from build123d import *

# Parameters (mm, degrees)
F0_W      = 44.5
F0_H      = 110
F0_R      = 2.65
F1_DEPTH  = 4
F2_W      = 44.5
F2_H      = 4
F3_DEPTH  = 20
F4_W      = 4
F4_H      = 68.5
F4_H_2    = 13.5
F5_DEPTH  = 20
F7_DEPTH  = 20
F9_DEPTH  = 15
F11_DEPTH = 44.501
F12_DEPTH = 20.001
F14_DEPTH = 20
F15_W     = 44.5
F15_H     = 9
F16_DEPTH = 1.5
F17_SIZE  = 1.49999
F18_DEPTH = 20.001
F19_SIZE  = 2


# Not quite as in the source:
# - a fillet or chamfer is up to 0.001 mm smaller than in the source, because OpenCascade refuses the exact size


with BuildPart() as f1:
    # F0 (on Top) → F1 (new body)
    with BuildSketch(Plane.XY):
        with Locations((22.25, 55)):
            Rectangle(F0_W, F0_H)
        with BuildLine():
            Line((25.25, 35), (25.25, 10))
            ThreePointArc((25.25, 10), (22.25, 7), (19.25, 10))
            Line((19.25, 10), (19.25, 35))
            ThreePointArc((19.25, 35), (22.25, 38), (25.25, 35))
        make_face(mode=Mode.SUBTRACT)
        with Locations((10, 100)):
            Circle(F0_R, mode=Mode.SUBTRACT)
        with Locations((22.25, 82.5)):
            Circle(F0_R, mode=Mode.SUBTRACT)
        with Locations((34.5, 100)):
            Circle(F0_R, mode=Mode.SUBTRACT)
    extrude(amount=F1_DEPTH)

    # F2 (on face) → F3 (join)
    with BuildSketch(Plane(origin=(0, 0, 0), x_dir=(1, 0, 0), z_dir=(0, 0, -1))):
        with Locations((22.25, -94.5)):
            Rectangle(F2_W, F2_H)
        with Locations((22.25, -70.5)):
            Rectangle(F2_W, F2_H)
    extrude(amount=F3_DEPTH)

    # F4 (on face) → F5 (join)
    with BuildSketch(Plane(origin=(0, 0, 0), x_dir=(1, 0, 0), z_dir=(0, 0, -1))):
        with Locations((2, -34.25)):
            Rectangle(F4_W, F4_H)
        with Locations((42.5, -34.25)):
            Rectangle(F4_W, F4_H)
        Polygon((0, -96.5), (0, -110), (4, -110), (4, -103.4641016151), (4, -96.5358983849), (4, -96.5), align=None)
        Polygon((4, -96.5358983849), (4, -103.4641016151), (10, -106.9282032303), (16, -103.4641016151), (16, -96.5358983849), (15.9378221735, -96.5), (11.9378221735, -96.5), (14, -97.6905989232), (14, -102.3094010768), (10, -104.6188021535), (6, -102.3094010768), (6, -97.6905989232), (8.0621778265, -96.5), (4.0621778265, -96.5), align=None)
        Polygon((11.9378221735, -96.5), (8.0621778265, -96.5), (6, -97.6905989232), (6, -102.3094010768), (10, -104.6188021535), (14, -102.3094010768), (14, -97.6905989232), align=None)
        Polygon((40.5, -110), (44.5, -110), (44.5, -96.5), (40.5, -96.5), (40.5, -96.5358983849), (40.5, -103.4641016151), align=None)
        Polygon((34.5, -106.9282032303), (40.5, -103.4641016151), (40.5, -96.5358983849), (40.4378221735, -96.5), (36.4378221735, -96.5), (38.5, -97.6905989232), (38.5, -102.3094010768), (34.5, -104.6188021535), (30.5, -102.3094010768), (30.5, -97.6905989232), (32.5621778265, -96.5), (28.5621778265, -96.5), (28.5, -96.5358983849), (28.5, -103.4641016151), align=None)
        Polygon((38.5, -97.6905989232), (36.4378221735, -96.5), (32.5621778265, -96.5), (30.5, -97.6905989232), (30.5, -102.3094010768), (34.5, -104.6188021535), (38.5, -102.3094010768), align=None)
        Polygon((32.5621778265, -96.5), (36.4378221735, -96.5), (34.5, -95.3811978465), align=None)
        with Locations((16.25, -34.25)):
            Rectangle(F4_W, F4_H)
        with Locations((28.25, -34.25)):
            Rectangle(F4_W, F4_H)
        with Locations((22.25, -103.25)):
            Rectangle(F4_W, F4_H_2)
    extrude(amount=F5_DEPTH)

    # F6 (on face) → F7 (join)
    with BuildSketch(Plane(origin=(0, 0, 0), x_dir=(1, 0, 0), z_dir=(0, 0, -1))):
        Polygon((40.5, -96.5), (40.4378221735, -96.5), (40.5, -96.5358983849), align=None)
        Polygon((4.0621778265, -96.5), (4, -96.5), (4, -96.5358983849), align=None)
        Polygon((16, -96.5358983849), (16, -103.4641016151), (20.25, -103.4641016151), (20.25, -96.5), (15.9378221735, -96.5), align=None)
        Polygon((28.5621778265, -96.5), (24.25, -96.5), (24.25, -103.4641016151), (28.5, -103.4641016151), (28.5, -96.5358983849), align=None)
    extrude(amount=F7_DEPTH)

    # F8 (on face) → F9 (cut)
    with BuildSketch(Plane(origin=(0, 0, -20), x_dir=(1, 0, 0), z_dir=(0, 0, -1))):
        Polygon((4, -103.4641016151), (10, -106.9282032303), (16, -103.4641016151), (20.25, -103.4641016151), (20.25, -96.5), (4, -96.5), align=None)
        Polygon((24.25, -103.4641016151), (28.5, -103.4641016151), (34.5, -106.9282032303), (40.5, -103.4641016151), (40.5, -96.5), (24.25, -96.5), align=None)
    extrude(amount=-F9_DEPTH, mode=Mode.SUBTRACT)

    # F10 (on face) → F11 (cut, through all)
    with BuildSketch(Plane(origin=(0, 0, 0), x_dir=(0, -1, 0), z_dir=(-1, 0, 0))):
        Polygon((-96.5, -20), (-110, 0), (-110, -20), align=None)
        Polygon((0, -5), (-68.5, -20), (0, -20), align=None)
    extrude(amount=-F11_DEPTH, mode=Mode.SUBTRACT)

    # F12 (cut, through all): faces of the model
    f12_faces = [f1.faces().sort_by_distance(p)[0] for p in [
        (34.5, 100, 0),
        (10, 100, 0),
    ]]
    extrude(f12_faces, amount=-F12_DEPTH, mode=Mode.SUBTRACT)

    # F13 (on face) → F14 (cut, through all)
    with BuildSketch(Plane(origin=(0, 0, -20), x_dir=(1, 0, 0), z_dir=(0, 0, -1))):
        Polygon((14, -102.3094010768), (14, -97.6905989232), (10, -95.3811978465), (6, -97.6905989232), (6, -102.3094010768), (10, -104.6188021535), align=None)
        Polygon((38.5, -102.3094010768), (38.5, -97.6905989232), (34.5, -95.3811978465), (30.5, -97.6905989232), (30.5, -102.3094010768), (34.5, -104.6188021535), align=None)
    extrude(amount=-F14_DEPTH, mode=Mode.SUBTRACT)

    # F15 (on face) → F16 (join)
    with BuildSketch(Plane(origin=(0, 0, 0), x_dir=(1, 0, 0), z_dir=(0, 0, -1))):
        with Locations((22.25, -82.5)):
            Rectangle(F15_W, F15_H)
    extrude(amount=F16_DEPTH)

    # F17 (size 1.5 in the source; OpenCascade refuses exactly that, so slightly less here)
    f17_edges = [f1.edges().sort_by_distance(p)[0] for p in [
        (44.5, 82.5, -1.5),
        (22.25, 78, -1.5),
        (0, 82.5, -1.5),
        (22.25, 87, -1.5),
    ]]
    chamfer(f17_edges, length=F17_SIZE)

    # F18 (cut, through all): a face of the model
    f18_faces = [f1.faces().sort_by_distance(p)[0] for p in [
        (22.25, 82.5, 0),
    ]]
    extrude(f18_faces, amount=-F18_DEPTH, mode=Mode.SUBTRACT)

    # F19
    f19_edges = [f1.edges().sort_by_distance(p)[0] for p in [
        (44.5, 110, 2),
        (0, 110, 2),
        (0, 0, -0.5),
        (44.5, 0, -0.5),
    ]]
    chamfer(f19_edges, length=F19_SIZE)


solid = f1.part
Check sheet for the modelled part. Datum: model origin and axes. Units: mm. A direction names the side the tool comes from. Give positions to 0.01 mm unless a question says otherwise; leave off trailing zeros. Order: outer loops, then holes, each group sorted by start corner. A loop starts at its lowest first (then second) coordinate and runs counter-clockwise, first axis right, second up. Notation, with made-up numbers: M -6.5,-11 L 47.5,-11 A24 ccw 47.5,6 Z; hole C 47.5,-11.75 d5. An arc over 180 degrees is marked long. Answer as CSV lines item,"result". Start each with the question number.
Item 1: Cross-section at B-B on y = 14.5. Enter the section's corners in (x, z), plus the area to 3 significant figures.
Item 2: Cross-section at A-A on x = 22.25. State how many separate pieces and enclosed holes the cut face has, plus the area to 3 significant figures.
Item 3: Gauge pin test, flat ends, axial feed: P1, Ø11, axis at x = 11.5, y = 103.5, coming from the -Z side; P2, Ø1.5, axis at x = 8, y = 63.5, coming from the -Z side; P3, Ø1.3, axis at x = 26.5, z = -2, coming from the +Y side; P4, Ø8, axis at y = 35, z = -17, coming from the +X side. Record the tip position at first contact, or that the pin passes through.
Item 4: Cross-section at D-D on y = 82.5. Enter the section's corners in (x, z).
Item 5: Mould release check, pull along Y, two halves, no side actions. Record for faces 1 (the face through (32.472, 103.448, -2.535)), 2 (the face through (22, 68.5, -10)), 3 (the face through (14, 103, -5)): +Y half, -Y half, draft (parallel to the pull), parting line (faces both ways), or undercut.
Item 6: Tool access check on faces 4 (the face through (28, 96.5, -13)), 5 (the face through (40.5, 42, -8)), 6 (the face through (11.97, 103.48, -2.54)), 7 (the face through (19.25, 22, 2)). Record the directions out of +Z, -Z, +X, -X, +Y, -Y that give a thin tool (end or side, any length) a straight path to the whole face; none if there is none.
Item 7: Thickness scan on line 1 (X direction, y = 32, z = -5.75); line 2 (Y direction, x = 22.5, z = 1.5); line 3 (Y direction, x = 25.5, z = -6.25). Record the ranges inside material, lowest first. Write a range as [from, to].
Established:
1,outline,"M 0,-8.18 L 4,-8.18 L 4,0 L 14.25,0 L 14.25,-8.18 L 18.25,-8.18 L 18.25,0 L 19.25,0 L 19.25,4 L 0,4 Z; M 25.25,0 L 26.25,0 L 26.25,-8.18 L 30.25,-8.18 L 30.25,0 L 40.5,0 L 40.5,-8.18 L 44.5,-8.18 L 44.5,4 L 25.25,4 Z"
1,area,"285 mm^2"
2,separate pieces,"3"
2,enclosed holes,"0"
2,area,"593 mm^2"
3,P1,"stops at z = -5"
3,P2,"stops at z = 0"
3,P3,"stops at y = 103.46"
3,P4,"passes through"
4,outline,"M 0,0 L 1.5,-1.5 L 19.6,-1.5 L 19.6,4 L 0,4 Z; M 24.9,-1.5 L 43,-1.5 L 44.5,0 L 44.5,4 L 24.9,4 Z"
5,face 1,"undercut"
5,face 2,"-Y half"
5,face 3,"draft"
6,face 4,"-Z, +Y"
6,face 5,"-Z, -Y"
6,face 6,"-Z"
6,face 7,"+Z, -Z"
7,line 1,"x = [0, 4], [14.25, 18.25], [26.25, 30.25], [40.5, 44.5]"
7,line 2,"y = [0, 7.01], [37.99, 79.86], [85.14, 110]"
7,line 3,"y = [68.5, 72.5], [92.5, 96.5]"
